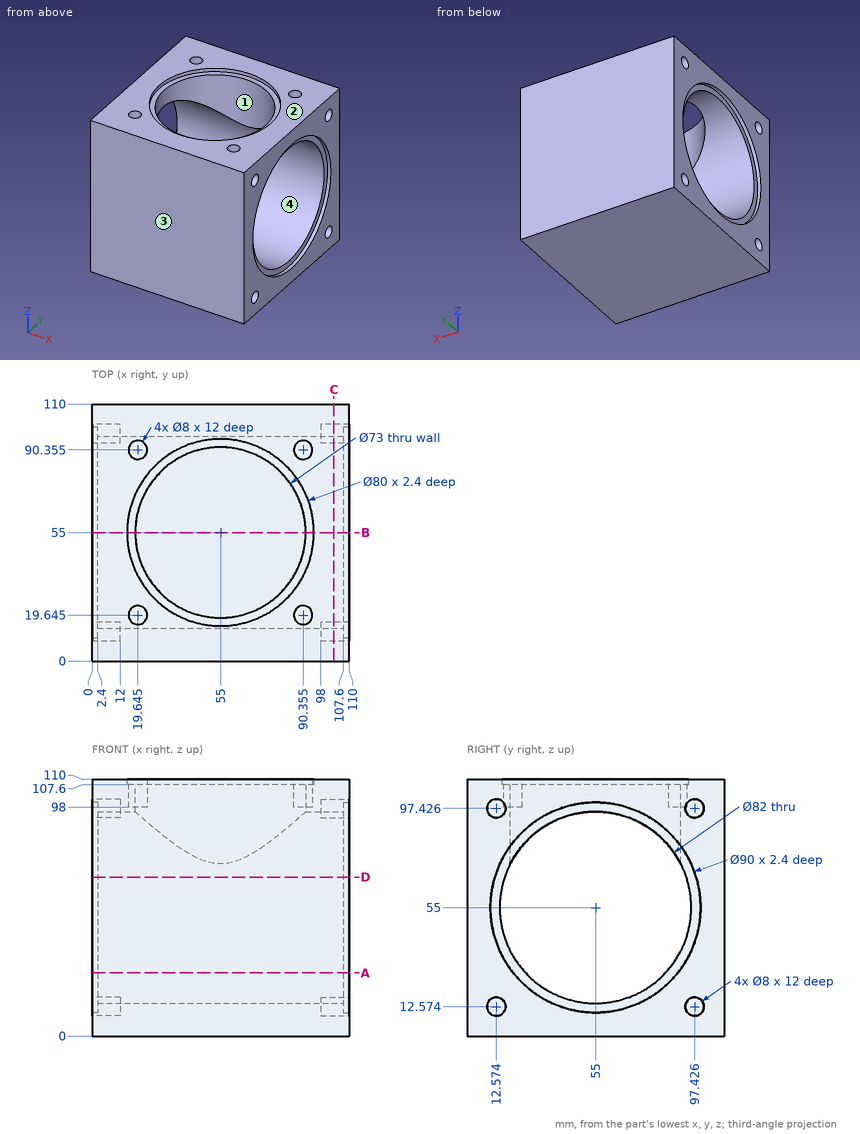
Drawing for the job (mm, zero at the part's lowest x, y, z). Give positions to 0.01 mm unless a question says otherwise; leave off trailing zeros. Write each loop counter-clockwise with the first axis right and the second up, starting at its lowest first coordinate (ties: lowest second). Pieces come first, ordered by that corner, then holes. Notation, with made-up numbers: M -25.75,24.25 L -20.75,24.25 A15 ccw -20.75,42.25 Z; hole C 86,45.5 d3. An arc over 180 degrees is marked long. Return JSON: item names as keys, results as strings. Group by question number.
(1) Band-saw the part on C-C (x = 103.5). Give the cut face in (y, z).
(2) Flat gauge pins, fed straight in: pin 1 Ø5 at (y, z) = (12.57, 97.43) entering from -X; pin 2 Ø4 at (y, z) = (13, 96.5) entering from +X. Where does each tip first touch, or does it go through?
(3) Band-saw the part on B-B (y = 55). Give the cut face in (x, z), and give its area (3 significant figures).
(4) Drill centre lines: L1, parallel to Y at x = 18, z = 22; L2, parallel to X at y = 56.5, z = 105.5; L3, parallel to Y at x = 49.5, z = 63.5. Where is each one in solid material? Low to high. Write a range as [from, to].
(5) Mould opens along Y. For the marked faces 1, 2, 3 and 4 say: pulls with the +Y half, pulls with the -Y half, needs draft (parallel to the pull), parting line crosses it, or undercut.
(6) Band-saw the part on D-D (z = 68). Give the cut face in (x, y) (1 decimal).
(7) Band-saw the part on A-A (z = 27). Give the cut face in (x, y), and give its area (3 significant figures).
Entries:
{
 "1": {"outline": "M 0,0 L 110,0 L 110,110 L 0,110 Z; hole C 12.57,12.57 d8; hole C 12.57,97.43 d8; hole C 55,55 d82; hole C 97.43,12.57 d8; hole C 97.43,97.43 d8"},
 "2": {"pin 1": "stops at x = 12", "pin 2": "stops at x = 98"},
 "3": {"outline": "M 0,0 L 110,0 L 110,10 L 107.6,10 L 107.6,14 L 2.4,14 L 2.4,10 L 0,10 Z; M 0,100 L 2.4,100 L 2.4,96 L 18.5,96 L 18.5,107.6 L 15,107.6 L 15,110 L 0,110 Z; M 91.5,96 L 107.6,96 L 107.6,100 L 110,100 L 110,110 L 95,110 L 95,107.6 L 91.5,107.6 Z", "area": "2,000 mm^2"},
 "4": {"L1": "y = [0, 30.67], [79.33, 110]", "L2": "x = [0, 18.53], [91.47, 110]", "L3": "y = [0, 14.89], [95.11, 110]"},
 "5": {"face 1": "undercut", "face 2": "needs draft", "face 3": "pulls with the -Y half", "face 4": "undercut"},
 "6": {"outline": "M 0,0 L 110,0 L 110,11.9 L 107.6,11.9 L 107.6,16.1 L 2.4,16.1 L 2.4,11.9 L 0,11.9 Z; M 0,98.1 L 2.4,98.1 L 2.4,93.9 L 107.6,93.9 L 107.6,98.1 L 110,98.1 L 110,110 L 0,110 Z"},
 "7": {"outline": "M 0,0 L 110,0 L 110,19.77 L 107.6,19.77 L 107.6,25.05 L 2.4,25.05 L 2.4,19.77 L 0,19.77 Z; M 0,90.23 L 2.4,90.23 L 2.4,84.95 L 107.6,84.95 L 107.6,90.23 L 110,90.23 L 110,110 L 0,110 Z", "area": "5,460 mm^2"}
}
